The model under review builds one solid part; all positions refer to its coordinate system, in mm. A direction names the side the tool comes from. Coordinates: 2 decimals unless noted, no trailing zeros. Order: outer loops, then holes, each group sorted by start corner. A loop starts at its lowest first (then second) coordinate and runs counter-clockwise, first axis right, second up.
```python
from build123d import *

# Parameters (mm, degrees)
SKETCH1_R           = 52.5
BOSS_EXTRUDE1_DEPTH = 7
SKETCH2_R           = 35
SKETCH2_R_2         = 31.83
BOSS_EXTRUDE3_DEPTH = 20
SKETCH3_R           = 3
CUT_EXTRUDE1_DEPTH  = 20
SKETCH4_R           = 5.25
CUT_EXTRUDE2_DEPTH  = 3
SKETCH5_W           = 10.2
SKETCH5_H           = 12.2
CUT_EXTRUDE3_DEPTH  = 120
BOSS_EXTRUDE4_START = -3
SKETCH6_R           = 31.83
BOSS_EXTRUDE4_DEPTH = 3


with BuildPart() as part:
    # Sketch1 → Boss-Extrude1 (new body)
    with BuildSketch(Plane(origin=(0, 0, 0), x_dir=(1, 0, 0), z_dir=(0, 1, 0))):
        with Locations(Location((0, 0, 0), (0, 0, 270))):
            Circle(SKETCH1_R)
    extrude(amount=BOSS_EXTRUDE1_DEPTH)

    # Sketch2 → Boss-Extrude3 (add)
    with BuildSketch(Plane(origin=(0, 7, 0), x_dir=(1, 0, 0), z_dir=(0, 1, 0))):
        with Locations(Location((0, 0, 0), (0, 0, 270))):
            Circle(SKETCH2_R)
        with Locations(Location((0, 0, 0), (0, 0, 270))):
            Circle(SKETCH2_R_2, mode=Mode.SUBTRACT)
    extrude(amount=BOSS_EXTRUDE3_DEPTH)

    # Sketch3 → Cut-Extrude1 (cut)
    with BuildSketch(Plane(origin=(0, 7, 0), x_dir=(1, 0, 0), z_dir=(0, 1, 0))):
        with Locations(Location((0, 46.25, 0), (0, 0, 270))):
            Circle(SKETCH3_R)
        with Locations(Location((46.25, 0, 0), (0, 0, 270))):
            Circle(SKETCH3_R)
        with Locations(Location((0, -46.25, 0), (0, 0, 270))):
            Circle(SKETCH3_R)
        with Locations(Location((-46.25, 0, 0), (0, 0, 270))):
            Circle(SKETCH3_R)
    extrude(amount=-CUT_EXTRUDE1_DEPTH, mode=Mode.SUBTRACT)

    # Sketch4 → Cut-Extrude2 (cut)
    with BuildSketch(Plane(origin=(0, 7, 0), x_dir=(1, 0, 0), z_dir=(0, 1, 0))):
        with Locations(Location((0, 46.25, 0), (0, 0, 270))):
            Circle(SKETCH4_R)
        with Locations(Location((46.25, 0, 0), (0, 0, 270))):
            Circle(SKETCH4_R)
        with Locations(Location((0, -46.25, 0), (0, 0, 270))):
            Circle(SKETCH4_R)
        with Locations(Location((-46.25, 0, 0), (0, 0, 270))):
            Circle(SKETCH4_R)
    extrude(amount=-CUT_EXTRUDE2_DEPTH, mode=Mode.SUBTRACT)

    # Sketch5 → Cut-Extrude3 (cut)
    with BuildSketch(Plane(origin=(60, 0, 0), x_dir=(0, 0, -1), z_dir=(1, 0, 0))):
        with Locations((0, 17)):
            Rectangle(SKETCH5_W, SKETCH5_H)
    extrude(amount=-CUT_EXTRUDE3_DEPTH, mode=Mode.SUBTRACT)

    # Sketch6 → Boss-Extrude4 (add)
    with BuildSketch(Plane(origin=(0, 27, 0), x_dir=(1, 0, 0), z_dir=(0, 1, 0)).offset(BOSS_EXTRUDE4_START)):
        with Locations(Location((0, 0, 0), (0, 0, 270))):
            Circle(SKETCH6_R)
    extrude(amount=BOSS_EXTRUDE4_DEPTH)


solid = part.part
```
(1) Draft analysis for pull direction Z (two halves, no side actions). For faces 5 (the face through (15.77, 3.451, 50.076)), 6 (the face through (-2.3, 4, -44)), 7 (the face through (0, 7, 0)), 8 (the face through (1, 0, -1)), state which applies: released by +Z, released by -Z, zero draft, split by the parting line, or undercut.
A:
face 5: split by the parting line
face 6: undercut
face 7: undercut
face 8: zero draft
(2) Machinability: for faces 1 (the face through (0.132, 2.028, -49.247)), 2 (the face through (-34, 7, 11)), 3 (the face through (33, 17, -5.1)), 4 (the face through (0, 24, 0)), which of the approach directions +Z, -Z, +X, -X, +Y, -Y give a long, thin tool a straight path to every point of the face, cutting with its end or side? Answer none if there is none.
A:
face 1: +Y, -Y
face 2: +Y
face 3: +X, -X
face 4: none
(3) For pin 1 Ø5 at (y, z) = (11.5, -29.5) entering from +X; pin 2 Ø1.6 at (x, y) = (32.5, 16.5) entering from -Z; pin 3 Ø8 at (y, z) = (21, 2.5) entering from -X, all flat-tipped, find the tip position at first contact; note any pin that passes through.
A:
pin 1: stops at x = 22.27
pin 2: stops at z = -14.84
pin 3: stops at x = -35
(4) We need section A-A, the plane y = 12.75. Write out the cut boundary in (x, z), and give its area (3 significant figures).
A:
outline: (-34.63, -5.1) arc R35 ccw to (34.63, -5.1) - (31.42, -5.1) arc R31.83 cw to (-31.42, -5.1) - close; (-34.63, 5.1) - (-31.42, 5.1) arc R31.83 cw to (31.42, 5.1) - (34.63, 5.1) arc R35 ccw to start
area: 601 mm2
(5) We need section D-D, the plane z = -46.25. Write out the cut boundary in (x, y), and give its area (3 significant figures).
A:
outline: (-24.84, 0) - (-3, 0) - (-3, 4) - (-5.25, 4) - (-5.25, 7) - (-24.84, 7) - close; (3, 0) - (24.84, 0) - (24.84, 7) - (5.25, 7) - (5.25, 4) - (3, 4) - close
area: 292 mm2
(6) We need section C-C, the plane x = 25.5. Write out the cut boundary in (y, z).
A:
outline: (0, -45.89) - (7, -45.89) - (7, -23.97) - (27, -23.97) - (27, 23.97) - (7, 23.97) - (7, 45.89) - (0, 45.89) - close; hole (7, -19.05) - (24, -19.05) - (24, 19.05) - (7, 19.05) - close
(7) Wall thickness on probe 1 along X at (y, z) = (4.95, 0); probe 2 along X at (y, z) = (0.8, 0); probe 3 along Y at (x, z) = (32.5, 3.5): over which ranges is each line inside the solid? List them lowest first.
A:
probe 1: x = -52.5 to -51.5, -41 to 41, 51.5 to 52.5
probe 2: x = -52.5 to -49.25, -43.25 to 43.25, 49.25 to 52.5
probe 3: y = 0 to 10.9, 23.1 to 27
(8) We need section B-B, the plane x = -46.25. Write out the cut boundary in (y, z).
A:
outline: (0, -24.84) - (7, -24.84) - (7, -5.25) - (4, -5.25) - (4, -3) - (0, -3) - close; (0, 3) - (4, 3) - (4, 5.25) - (7, 5.25) - (7, 24.84) - (0, 24.84) - close
